from build123d import *

# Parameters (mm, degrees)
SKETCH3_W           = 70
SKETCH3_H           = 50
SKETCH3_R           = 4
BOSS_EXTRUDE1_DEPTH = 7.5
SKETCH4_W           = 70
SKETCH4_H           = 7.5
BOSS_EXTRUDE2_DEPTH = 20
FILLET3_R           = 10


with BuildPart() as part:
    # Sketch3 → Boss-Extrude1 (new body)
    with BuildSketch(Plane(origin=(0, 0, 0), x_dir=(1, 0, 0), z_dir=(0, 1, 0))):
        with Locations((4.469051839, 0.071060676)):
            Rectangle(SKETCH3_W, SKETCH3_H)
        with Locations(Location((32.469051839, 0.071060676, 0), (0, 0, 270))):
            Circle(SKETCH3_R, mode=Mode.SUBTRACT)
        with Locations(Location((-23.530948161, 0.071060676, 0), (0, 0, 90))):
            Circle(SKETCH3_R, mode=Mode.SUBTRACT)
    extrude(amount=BOSS_EXTRUDE1_DEPTH)

    # Sketch4 → Boss-Extrude2 (add)
    with BuildSketch(Plane(origin=(0, 7.5, 0), x_dir=(1, 0, 0), z_dir=(0, 1, 0))):
        with Locations((4.469051839, 21.321060676)):
            Rectangle(SKETCH4_W, SKETCH4_H)
    extrude(amount=BOSS_EXTRUDE2_DEPTH)

    # Fillet3
    fillet3_edges = [part.edges().sort_by_distance(p)[0] for p in [
        (4.469051839, 7.5, -17.571060676),
    ]]
    fillet(fillet3_edges, radius=FILLET3_R)


solid = part.part
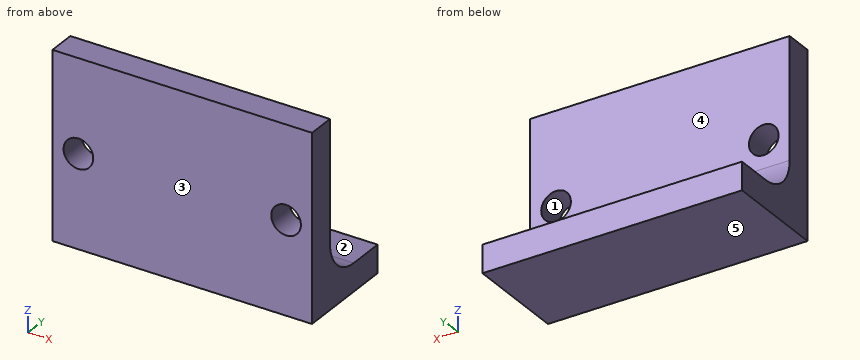
Model file for the job. Use its own axes, mm. Face numbers are marked on the shaded views. A direction names the side the tool comes from. Give positions to 0.01 mm unless a question says otherwise; leave off trailing zeros. Order: outer loops, then holes, each group sorted by start corner. A loop starts at its lowest first (then second) coordinate and runs counter-clockwise, first axis right, second up. Notation, with made-up numbers: (23, -11.5) - (51, -11.5) arc R17 ccw to (51, -5.5) - close; hole circle Ø9 at (28, -6.5). An arc over 180 degrees is marked (long way). Write item = value, one per line. Start each with the question number.
1. Which spindle directions (+Z, -Z, +X, -X, +Y, -Y) get a long thin tool onto all of the face, cutting with end or side? Do the marked faces 4 and 5. Say none if no direction does.
2. Cut at C-C, the plane y = 3.75. List the corners of the cut face in (x, z).
3. Cut at D-D, the plane y = 23. List the corners of the cut face in (x, z), and give its area (3 significant figures).
4. Cut at B-B, the plane z = 3. List the corners of the cut face in (x, y).
5. Probe line 1 along Z through (x, y) = (-12, 21.25); line 2 along Y through (x, z) = (1, 22); line 3 along Y through (x, z) = (0.5, -15). List the from-to ranges inside material, lowest first.
6. Cut at A-A, the plane x = 14.5. List the corners of the cut face in (y, z), and give its area (3 significant figures).
7. Drop flat-ended pins along their axis: P1, Ø3, axis at x = 14, y = 21.5, coming from the +Z side; P2, Ø10, axis at x = 5.5, z = 12.5, coming from the +Y side. Give the stop position or say it passes through.
8. Two-plate mould, pull along Z, no slides. Class the marked faces 1, 2 and 3: pulls with the +Z half, pulls with the -Z half, needs draft (parallel to the pull), parting line crosses it, or undercut.
Taken from the geometry:
q1.face_4 = +Z, +X, -X, +Y
q1.face_5 = -Z, +X, -X, +Y, -Y
q2.outline = (-30.53, -25.07) - (39.47, -25.07) - (39.47, 24.93) - (-30.53, 24.93) - close; hole circle Ø8 at (-23.53, -0.07); hole circle Ø8 at (32.47, -0.07)
q3.outline = (-30.53, -25.07) - (39.47, -25.07) - (39.47, -17.57) - (-30.53, -17.57) - close
q3.area = 525 mm²
q4.outline = (-30.53, 0) - (-26.09, 0) - (-26.09, 7.5) - (-30.53, 7.5) - close; (-20.97, 0) - (29.91, 0) - (29.91, 7.5) - (-20.97, 7.5) - close; (35.03, 0) - (39.47, 0) - (39.47, 7.5) - (35.03, 7.5) - close
q5.line_1 = -25.07 to -17.57
q5.line_2 = 0 to 7.5
q5.line_3 = 0 to 10.81
q6.outline = (0, -25.07) - (27.5, -25.07) - (27.5, -17.57) - (17.5, -17.57) arc R10 cw to (7.5, -7.57) - (7.5, 24.93) - (0, 24.93) - close
q6.area = 546 mm²
q7.P1 = -17.57
q7.P2 = 7.5
q8.face_1 = undercut
q8.face_2 = pulls with the +Z half
q8.face_3 = needs draft
